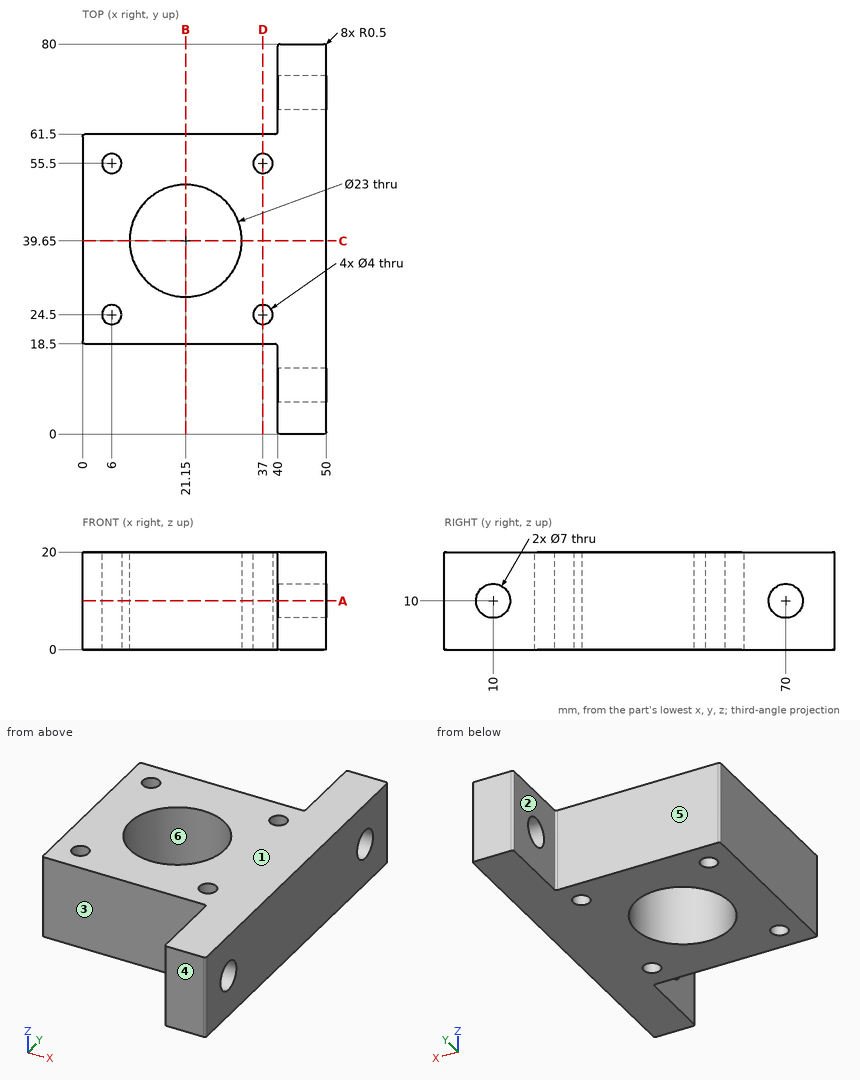
Check sheet for the drawn part. Datum: minimum x, y, z corner. Units: mm. A direction names the side the tool comes from. Round coordinates to 2 decimals unless told otherwise and drop trailing zeros. Write each loop counter-clockwise with the first axis right and the second up, starting at its lowest first coordinate (ties: lowest second). Pieces come first, ordered by that corner, then holes. Notation, with made-up numbers: (69.5, -34) -> (113.5, -34) arc R17 cw to (113.5, -13) -> close; hole circle Ø7 at (-35, 0.25). An arc over 180 degrees is marked (long way). Put each result on its own line as item: value.
(1) Material ranges on line 1 (Y direction, x = 37, z = 10.5); line 2 (X direction, y = 24.5, z = 7.25); line 3 (X direction, y = 55, z = 8.75), recorded low to high.
Values found:
line 1: y = 18.5 to 22.5, 26.5 to 53.5, 57.5 to 61.5
line 2: x = 0 to 4, 8 to 35, 39 to 50
line 3: x = 0 to 4.06, 7.94 to 35.06, 38.94 to 50
(2) Sectioned sample at D-D (x = 37). Enter the section's corners in (y, z).
Values found:
outline: (18.5, 0) -> (22.5, 0) -> (22.5, 20) -> (18.5, 20) -> close; (26.5, 0) -> (53.5, 0) -> (53.5, 20) -> (26.5, 20) -> close; (57.5, 0) -> (61.5, 0) -> (61.5, 20) -> (57.5, 20) -> close
(3) Mould release check, pull along Y, two halves, no side actions. Record for the marked faces 4, 5 and 6: released by +Y, released by -Y, zero draft, split by the parting line, or undercut.
Values found:
face 4: released by -Y
face 5: released by +Y
face 6: undercut
(4) Tool access check on the marked faces 1, 2 and 3. Record the directions out of +Z, -Z, +X, -X, +Y, -Y that give a thin tool (end or side, any length) a straight path to the whole face; none if there is none.
Values found:
face 1: +Z, +X, -X, +Y, -Y
face 2: +Z, -Z, -X, +Y
face 3: +Z, -Z, -X, -Y
(5) Go/stop test with flat-tipped pins: pin 1 Ø8 at (x, z) = (33.5, 16) entering from -Y; pin 2 Ø9 at (y, z) = (68, 12.5) entering from -X. Record where each tip stops, or that it passes through.
Values found:
pin 1: stops at y = 18.5
pin 2: stops at x = 40
(6) Sectioned sample at B-B (x = 21.15). Enter the section's corners in (y, z).
Values found:
outline: (18.5, 0) -> (28.15, 0) -> (28.15, 20) -> (18.5, 20) -> close; (51.15, 0) -> (61.5, 0) -> (61.5, 20) -> (51.15, 20) -> close
(7) Sectioned sample at A-A (z = 10). Count the separate pieces of the cut face and the enclosed holes in it, plus the area to 3 significant figures.
Values found:
separate pieces: 3
enclosed holes: 5
area: 1,910 mm^2
(8) Sectioned sample at C-C (y = 39.65). Enter the section's corners in (x, z), plus the area to 3 significant figures.
Values found:
outline: (0, 0) -> (9.65, 0) -> (9.65, 20) -> (0, 20) -> close; (32.65, 0) -> (50, 0) -> (50, 20) -> (32.65, 20) -> close
area: 540 mm^2
